from build123d import *

# Parameters (mm, degrees)
SKETCH1_W           = 4.5
SKETCH1_H           = 15.4
BOSS_EXTRUDE1_DEPTH = 33
CUT_EXTRUDE1_DEPTH  = 20
SKETCH2_4_W         = 7.347569662
SKETCH2_4_H         = 15
SKETCH2_4_W_2       = 0.152430338
CUT_EXTRUDE2_DEPTH  = 20
FILLET1_R           = 10
SKETCH3_R           = 1.5
CUT_EXTRUDE3_DEPTH  = 7
SKETCH3_3_R         = 1.5
CUT_EXTRUDE4_DEPTH  = 7
SKETCH3_4_R         = 1.5
BOSS_EXTRUDE2_DEPTH = 10
SKETCH3_5_R         = 1.5
CUT_EXTRUDE5_DEPTH  = 8
FILLET9_R           = 3
SKETCH20_W          = 10
SKETCH20_H          = 3
CUT_EXTRUDE6_DEPTH  = 25
FILLET10_R          = 3
FILLET11_R          = 10
FILLET12_R          = 3
FILLET13_R          = 3
CUT_EXTRUDE7_DEPTH  = 5
FILLET17_R          = 7.5
FILLET18_R          = 7.5
FILLET19_R          = 7.5


with BuildPart() as part:
    # Sketch1 → Boss-Extrude1 (new body)
    with BuildSketch(Plane(origin=(0, 0, 0), x_dir=(1, 0, 0), z_dir=(0, 1, 0))):
        Polygon((-4.5, 0.152430338), (0, 0.152430338), (0, 15.552430338), (4.5, 15.552430338), (4.5, 30), (-4.5, 30), align=None)
        with Locations((2.25, 7.852430338)):
            Rectangle(SKETCH1_W, SKETCH1_H)
        with BuildLine():
            ThreePointArc((-4.5, 0.152430338), (-2.251290464, 0.03811851), (0, 0))
            Line((0, 0), (0, 0.152430338))
            Line((0, 0.152430338), (-4.5, 0.152430338))
        make_face()
        with BuildLine():
            Line((0, 0.152430338), (0, 0))
            ThreePointArc((0, 0), (2.251290464, 0.03811851), (4.5, 0.152430338))
            Line((4.5, 0.152430338), (0, 0.152430338))
        make_face()
    extrude(amount=-BOSS_EXTRUDE1_DEPTH)

    # Sketch2 → Cut-Extrude1 (cut)
    with BuildSketch(Plane(origin=(4.5, 0, 0), x_dir=(0, 0, -1), z_dir=(1, 0, 0))):
        with BuildLine():
            ThreePointArc((18.727430338, -25.5), (17.797494369, -23.25493597), (15.552430338, -22.325))
            Line((15.552430338, -22.325), (15.552430338, -25.5))
            Line((15.552430338, -25.5), (15.552430338, -28.675))
            ThreePointArc((15.552430338, -28.675), (17.797494369, -27.74506403), (18.727430338, -25.5))
        make_face()
        with BuildLine():
            Line((15.552430338, -25.5), (15.552430338, -22.325))
            ThreePointArc((15.552430338, -22.325), (12.377430338, -25.5), (15.552430338, -28.675))
            Line((15.552430338, -28.675), (15.552430338, -25.5))
        make_face()
    extrude(amount=-CUT_EXTRUDE1_DEPTH, mode=Mode.SUBTRACT)

    # Sketch2_4 → Cut-Extrude2 (cut)
    with BuildSketch(Plane(origin=(4.5, 0, 0), x_dir=(0, 0, -1), z_dir=(1, 0, 0))):
        with Locations((3.826215169, -25.5)):
            Rectangle(SKETCH2_4_W, SKETCH2_4_H)
        with Locations((0.076215169, -25.5)):
            Rectangle(SKETCH2_4_W_2, SKETCH2_4_H)
        Polygon((0.152430338, -18), (7.5, -18), (0.152430338, -8.203240451), align=None)
        Polygon((0, -18), (0.152430338, -18), (0.152430338, -8.203240451), (0, -8), align=None)
    extrude(amount=-CUT_EXTRUDE2_DEPTH, mode=Mode.SUBTRACT)

    # Fillet1
    fillet1_edges = [part.edges().sort_by_distance(p)[0] for p in [
        (0, -33, -7.5),
    ]]
    fillet(fillet1_edges, radius=FILLET1_R)

    # Sketch3 → Cut-Extrude3 (cut)
    with BuildSketch(Plane(origin=(0, 0, 0), x_dir=(1, 0, 0), z_dir=(0, 1, 0))):
        with Locations(Location((0, 24.36613165, 0), (0, 0, 270))):
            Circle(SKETCH3_R)
    extrude(amount=-CUT_EXTRUDE3_DEPTH, mode=Mode.SUBTRACT)

    # Sketch3_3 → Cut-Extrude4 (cut)
    with BuildSketch(Plane(origin=(0, 0, 0), x_dir=(1, 0, 0), z_dir=(0, 1, 0))):
        with Locations(Location((0, 8.6922633, 0), (0, 0, 270))):
            Circle(SKETCH3_3_R)
    extrude(amount=-CUT_EXTRUDE4_DEPTH, mode=Mode.SUBTRACT)

    # Sketch3_4 → Boss-Extrude2 (add)
    # profile 1 of 6: a face of its own
    with BuildSketch(Plane(origin=(0, 0, 0), x_dir=(1, 0, 0), z_dir=(0, 1, 0))):
        Polygon((-14.5, 5.0022633), (-4.5, 5.0022633), (-4.5, 8.6922633), (-4.5, 12.3822633), (-4.5, 18.7322633), (-4.5, 30), (-14.5, 30), align=None)
        with Locations((-9.5, 8.6922633)):
            Circle(SKETCH3_4_R, mode=Mode.SUBTRACT)
        with Locations((-9.5, 24.36613165)):
            Circle(SKETCH3_4_R, mode=Mode.SUBTRACT)
    # profile 2 of 6: a face of its own
    with BuildSketch(Plane(origin=(0, 0, 0), x_dir=(1, 0, 0), z_dir=(0, 1, 0))):
        Polygon((4.5, 8.6922633), (4.5, 5.0022633), (14.5, 5.0022633), (14.5, 30), (4.5, 30), (4.5, 18.7322633), (4.5, 12.3822633), align=None)
        with Locations((9.5, 8.6922633)):
            Circle(SKETCH3_4_R, mode=Mode.SUBTRACT)
        with Locations((9.5, 24.36613165)):
            Circle(SKETCH3_4_R, mode=Mode.SUBTRACT)
    # profile 3 of 6: a face of its own
    with BuildSketch(Plane(origin=(0, 0, 0), x_dir=(1, 0, 0), z_dir=(0, 1, 0))):
        with Locations((-9.5, 24.36613165)):
            Circle(SKETCH3_4_R)
    # profile 4 of 6: a face of its own
    with BuildSketch(Plane(origin=(0, 0, 0), x_dir=(1, 0, 0), z_dir=(0, 1, 0))):
        with Locations((9.5, 24.36613165)):
            Circle(SKETCH3_4_R)
    # profile 5 of 6: a face of its own
    with BuildSketch(Plane(origin=(0, 0, 0), x_dir=(1, 0, 0), z_dir=(0, 1, 0))):
        with Locations((-9.5, 8.6922633)):
            Circle(SKETCH3_4_R)
    # profile 6 of 6: a face of its own
    with BuildSketch(Plane(origin=(0, 0, 0), x_dir=(1, 0, 0), z_dir=(0, 1, 0))):
        with Locations((9.5, 8.6922633)):
            Circle(SKETCH3_4_R)
    extrude(amount=-BOSS_EXTRUDE2_DEPTH)

    # Sketch3_5 → Cut-Extrude5 (cut)
    with BuildSketch(Plane(origin=(0, 0, 0), x_dir=(1, 0, 0), z_dir=(0, 1, 0))):
        with Locations(Location((-9.5, 8.6922633, 0), (0, 0, 270))):
            Circle(SKETCH3_5_R)
        with Locations(Location((9.5, 8.6922633, 0), (0, 0, 270))):
            Circle(SKETCH3_5_R)
        with Locations(Location((9.5, 24.36613165, 0), (0, 0, 270))):
            Circle(SKETCH3_5_R)
        with Locations(Location((-9.5, 24.36613165, 0), (0, 0, 270))):
            Circle(SKETCH3_5_R)
    extrude(amount=-CUT_EXTRUDE5_DEPTH, mode=Mode.SUBTRACT)

    # Fillet9
    fillet9_edges = [part.edges().sort_by_distance(p)[0] for p in [
        (-2.253575518, -8.050927935, -0.038195951),
        (0, -18, -7.5),
    ]]
    fillet(fillet9_edges, radius=FILLET9_R)

    # Sketch20 → Cut-Extrude6 (cut)
    with BuildSketch(Plane.XY.offset(-5.0022633)):
        with Locations((-9.5, -8.5)):
            Rectangle(SKETCH20_W, SKETCH20_H)
        with Locations((9.5, -8.5)):
            Rectangle(SKETCH20_W, SKETCH20_H)
    extrude(amount=-CUT_EXTRUDE6_DEPTH, mode=Mode.SUBTRACT)

    # Fillet10
    fillet10_edges = [part.edges().sort_by_distance(p)[0] for p in [
        (4.5, -3.5, -5.0022633),
        (-4.5, -3.5, -5.0022633),
    ]]
    fillet(fillet10_edges, radius=FILLET10_R)

    # Fillet11
    fillet11_edges = [part.edges().sort_by_distance(p)[0] for p in [
        (0, -33, -30),
    ]]
    fillet(fillet11_edges, radius=FILLET11_R)

    # Fillet12
    fillet12_edges = [part.edges().sort_by_distance(p)[0] for p in [
        (14.5, -3.5, -5.0022633),
        (14.5, -3.5, -30),
        (-14.5, -3.5, -5.0022633),
        (-14.5, -3.5, -30),
    ]]
    fillet(fillet12_edges, radius=FILLET12_R)

    # Fillet13
    fillet13_edges = [part.edges().sort_by_distance(p)[0] for p in [
        (4.5, -7, -16.00113165),
        (-4.5, -7, -16.00113165),
    ]]
    fillet(fillet13_edges, radius=FILLET13_R)

    # Sketch21 → Cut-Extrude7 (cut, symmetric)
    with BuildSketch(Plane(origin=(0, 0, 0), x_dir=(0, 0, -1), z_dir=(1, 0, 0))):
        Polygon((31.193881394, -32.39723809), (31.193881394, -10), (30, -10), (23.419344423, -18.511746958), (23.419344423, -32.39723809), align=None)
        Polygon((23.419344423, -32.39723809), (23.419344423, -31.964785254), (7.776068465, -31.964785254), (7.488922124, -35.386612487), (23.419344423, -35.386612487), align=None)
    extrude(amount=CUT_EXTRUDE7_DEPTH, both=True, mode=Mode.SUBTRACT)

    # Fillet17
    fillet17_edges = [part.edges().sort_by_distance(p)[0] for p in [
        (0, -31.964785254, -23.419344423),
    ]]
    fillet(fillet17_edges, radius=FILLET17_R)

    # Fillet18
    fillet18_edges = [part.edges().sort_by_distance(p)[0] for p in [
        (0, -31.964785254, -13.069128149),
    ]]
    fillet(fillet18_edges, radius=FILLET18_R)

    # Fillet19
    fillet19_edges = [part.edges().sort_by_distance(p)[0] for p in [
        (0, -18.511746958, -23.419344423),
        (0, -10, -30),
    ]]
    fillet(fillet19_edges, radius=FILLET19_R)


solid = part.part
Work out the finished part from the listing and answer in its coordinate system (mm). A direction names the side the tool comes from. Give positions to 0.01 mm unless a question says otherwise; leave off trailing zeros. Write each loop counter-clockwise with the first axis right and the second up, starting at its lowest first coordinate (ties: lowest second). Pieces come first, ordered by that corner, then holes. Notation, with made-up numbers: (47, 31.5) - (91, 31.5) arc R27 ccw to (91, 61.5) - close; hole circle Ø9 at (-35.75, 6). An arc over 180 degrees is marked (long way). One line per item, written item: value. Start each with the question number.
1. Given pin 1 (0.9 mm diameter, centred on x = 0, z = -23.5, fed in from +Y); pin 2 (5.5 mm diameter, centred on x = -11, z = -16.5, fed in from -Y); pin 3 (3 mm diameter, centred on x = -10, y = -3, fed in from +Z), each flat-ended and moving along its own axis, determine where each tip first touches the part or whether it passes through.
2. Find section B-B (y = -2.5). Write down the section's boundary in (x, z), then the cut area to 3 significant figures.
3. For a pull along X with two mould halves and no side action, classify faces 4 (the cylindrical face through (9.57, -3.45, -10.19)), 5 (the cylindrical face through (5.4, -7.86, -15.81)), 6 (the flat face through (9, -3, -5.002)) as +X half, -X half, draft (parallel to the pull), parting line (faces both ways), or undercut.
4. For faces 1 (the flat face through (11, -7, -17)), 2 (the cylindrical face through (0.07, -3.45, -10.19)), 3 (the flat face through (0, -23, -23.419)), determine the directions among +Z, -Z, +X, -X, +Y, -Y from which every point of the face is accessible in a straight line to the end or side of a thin tool.
5. Find section A-A (x = 9.5). Write down the section's boundary in (y, z).
6. Consider probe 1 along X at (y, z) = (-4.5, -24); probe 2 along X at (y, z) = (-18.5, -15); probe 3 along Y at (x, z) = (-8.25, -22). Determine where each line is inside the solid, lowest interval first.
7. Find section D-D (y = -26). Write down the section's boundary in (x, z), then the cut area to 3 significant figures.
8. Find section C-C (z = -15). Write down the section's boundary in (x, y).
Geometry results:
1. pin 1: y = -7
1. pin 2: y = -7
1. pin 3: z = -5
2. outline: (-14.5, -27) arc R3 ccw to (-11.5, -30) - (11.5, -30) arc R3 ccw to (14.5, -27) - (14.5, -8) arc R3 ccw to (11.5, -5) - (7.5, -5) arc R3 cw to (4.5, -2) - (4.5, -0.15) arc R66.5 ccw to (-4.5, -0.15) - (-4.5, -2) arc R3 cw to (-7.5, -5) - (-11.5, -5) arc R3 ccw to (-14.5, -8) - close; hole circle Ø3 at (-9.5, -24.37); hole circle Ø3 at (-9.5, -8.69); hole circle Ø3 at (0, -24.37); hole circle Ø3 at (0, -8.69); hole circle Ø3 at (9.5, -24.37); hole circle Ø3 at (9.5, -8.69)
2. area: 723 mm2
3. face 4: undercut
3. face 5: +X half
3. face 6: draft
4. face 1: +Z, -Z, +X, -Y
4. face 2: +Y
4. face 3: -Z, +X, -X, -Y
5. outline: (-7, -30) - (0, -30) - (0, -25.87) - (-7, -25.87) - close; (-7, -22.87) - (0, -22.87) - (0, -10.19) - (-7, -10.19) - close; (-7, -7.19) - (0, -7.19) - (0, -5) - (-7, -5) - close
6. probe 1: -14.5 to -10.95, -8.05 to -1.45, 1.45 to 8.05, 10.95 to 14.5
6. probe 2: -4.5 to 4.5
6. probe 3: -7 to 0
7. outline: (-4.5, -23.26) - (4.5, -23.26) - (4.5, -18.69) - (-4.5, -18.69) - close; (-4.5, -12.42) - (4.5, -12.42) - (4.5, -7.96) - (-4.5, -7.96) - close
7. area: 81.3 mm2
8. outline: (-14.5, -7) - (-7.5, -7) arc R3 cw to (-4.5, -10) - (-4.5, -22.37) - (4.5, -22.37) - (4.5, -10) arc R3 cw to (7.5, -7) - (14.5, -7) - (14.5, 0) - (-14.5, 0) - close; (-4.5, -31.95) - (4.5, -31.95) - (4.5, -28.63) - (-4.5, -28.63) - close
